Input: part model. Units: mm. Frame: model coordinates. Face numbers are marked on the shaded views. A direction names the side the tool comes from. Give positions to 0.01 mm unless a question says otherwise; leave off trailing zeros. Loops run counter-clockwise (first coordinate to the right, second up) from the corner with the lowest first, then second, coordinate; pieces in that order, holes last. Notation, with made-up numbers: (49.25, 51) - (107.25, 51) arc R8 ccw to (107.25, 58) - close; hole circle Ø7 at (-4.5, 5). An arc over 180 degrees is marked (long way). One line per question, with ' | ' between items. Start each with the question number.
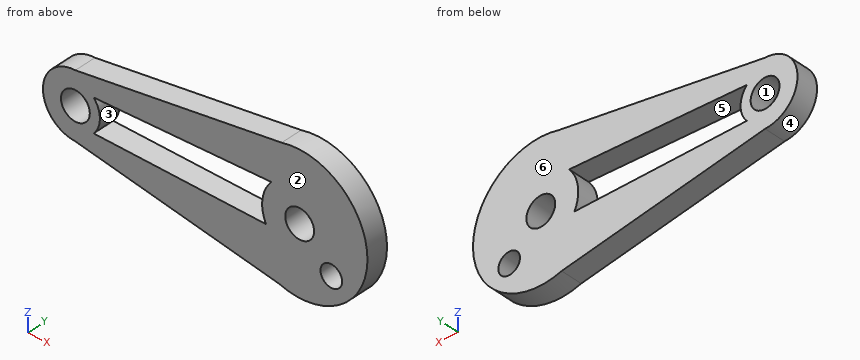
from build123d import *

# Parameters (mm, degrees)
SKETCH1_R           = 2
SKETCH1_R_2         = 1.5
BOSS_EXTRUDE1_DEPTH = 3


with BuildPart() as part:
    # Sketch1 → Boss-Extrude1 (new body)
    with BuildSketch(Plane(origin=(0, 0, 0), x_dir=(1, 0, 0), z_dir=(0, 1, 0))):
        with BuildLine():
            Line((-51.730151438, -5.002739553), (-23.52046035, -0.558125845))
            ThreePointArc((-23.52046035, -0.558125845), (-11.232359056, -9.299028138), (-23.130151438, -18.56419639))
            Line((-23.130151438, -18.56419639), (-51.730151438, -14.002739553))
            ThreePointArc((-51.730151438, -14.002739553), (-56.230151438, -9.502739553), (-51.730151438, -5.002739553))
        make_face()
        with Locations(Location((-20.630151438, -9.502739553, 0), (0, 0, 270))):
            Circle(SKETCH1_R, mode=Mode.SUBTRACT)
        with Locations(Location((-51.730151438, -9.502739553, 0), (0, 0, 270))):
            Circle(SKETCH1_R, mode=Mode.SUBTRACT)
        with Locations(Location((-16.247019321, -5.002739553, 0), (0, 0, 270))):
            Circle(SKETCH1_R_2, mode=Mode.SUBTRACT)
        with BuildLine():
            Line((-49.20201043, -7.229305358), (-25.30201043, -7.219379406))
            ThreePointArc((-25.30201043, -7.219379406), (-25.78692763, -10.171813025), (-24.564614553, -12.902739553))
            Line((-24.564614553, -12.902739553), (-49.20201043, -11.776173749))
            ThreePointArc((-49.20201043, -11.776173749), (-48.330151438, -9.502739553), (-49.20201043, -7.229305358))
        make_face(mode=Mode.SUBTRACT)
    extrude(amount=BOSS_EXTRUDE1_DEPTH)


solid = part.part
Q1. Access query for the marked faces 5 and 6. Directions: +Z, -Z, +X, -X, +Y, -Y. A direction counts if a zero-diameter tool reaches every point of the face in a straight line with its end or side. Return the directions, or none.
Q2. First-contact query: pin 1 (1.5 mm diameter, centred on x = -33, y = 2, fed in from +Z); pin 2 (1.5 mm diameter, centred on y = 1, z = 10.5, fed in from +X). Flat tips, straight axial feed; report the tip coordinate or a pass-through.
Q3. Draft query along X for the marked faces 1, 2, 3 and 4. Return one class per face: +X half, -X half, draft (parallel to the pull), parting line (faces both ways), or undercut.
Q4. Section D-D, the plane y = 1.3. Output: boundary loops of the cut face in (x, z), plus the area to 3 significant figures.
Q5. Line query: L1, parallel to X at y = 0.7, z = 11.25; L2, parallel to X at y = 0.2, z = 9.5; L3, parallel to Z at x = -25, y = 1.4. Output: solid intervals per line, ascending. Write a range as from..to.
Q6. Section A-A, the plane x = -15.5. Output: boundary loops of the cut face in (y, z).
Q7. Section B-B, the plane z = 9.25. Output: boundary loops of the cut face in (x, y).
Q8. Section C-C, the plane z = 4.25. Output: boundary loops of the cut face in (x, y).
Solved:
1) face 5: +Y, -Y | face 6: +Z, -Z, +X, -X, +Y
2) pin 1: stops at z = 17.11 | pin 2: stops at x = -11.23
3) face 1: undercut | face 2: draft | face 3: undercut | face 4: -X half
4) outline: (-51.73, 5) - (-23.52, 0.56) arc R9.4 ccw (long way) to (-23.13, 18.56) - (-51.73, 14) arc R4.5 ccw to start; hole circle Ø4 at (-51.73, 9.5); hole (-49.2, 7.23) - (-25.3, 7.22) arc R5.2 cw to (-24.56, 12.9) - (-49.2, 11.78) arc R3.4 cw to start; hole circle Ø4 at (-20.63, 9.5); hole circle Ø3 at (-16.25, 5) | area: 454 mm²
5) L1: x = -55.88..-52.7, -50.76..-48.81, -25.53..-21.6, -19.66..-11.39 | L2: x = -56.23..-53.73, -49.73..-48.33, -25.83..-22.63, -18.63..-11.23 | L3: z = 0.79..12.32, 12.88..18.27
6) outline: (0, 1.63) - (3, 1.63) - (3, 3.7) - (0, 3.7) - close; (0, 6.3) - (3, 6.3) - (3, 17.38) - (0, 17.38) - close
7) outline: (-56.22, 0) - (-53.71, 0) - (-53.71, 3) - (-56.22, 3) - close; (-49.75, 0) - (-48.34, 0) - (-48.34, 3) - (-49.75, 3) - close; (-25.82, 0) - (-22.61, 0) - (-22.61, 3) - (-25.82, 3) - close; (-18.65, 0) - (-11.23, 0) - (-11.23, 3) - (-18.65, 3) - close
8) outline: (-46.95, 0) - (-17.54, 0) - (-17.54, 3) - (-46.95, 3) - close; (-14.95, 0) - (-12.83, 0) - (-12.83, 3) - (-14.95, 3) - close
